```python
from build123d import *

# Parameters (mm, degrees)
F0_R     = 15.9266250138
F0_R_2   = 6.35
F1_DEPTH = 50.8
F2_R     = 3.4266006547
F3_DEPTH = 50.8
F7_R     = 6.4098114124
F8_DEPTH = 76.2


with BuildPart() as f1:
    # F0 (on Top) → F1 (new body)
    with BuildSketch(Plane.XY):
        Circle(F0_R)
        Circle(F0_R_2, mode=Mode.SUBTRACT)
    extrude(amount=F1_DEPTH)



with BuildPart() as f3:
    # F2 (on Top) → F3 (new body)
    with BuildSketch(Plane.XY):
        with Locations((-12.2786890715, 12.5171002001)):
            Circle(F2_R)
    extrude(amount=F3_DEPTH)


with BuildPart() as f4_1:
    # F4: copy of F3
    add(f3.part.moved(Location((24.45152, 0, 0))))


with BuildPart() as f5_1:
    # F5: copy of F4_1
    add(f4_1.part.moved(Location((0, -25.53886, 0))))


with BuildPart() as f6_1:
    # F6: copy of F5_1
    add(f5_1.part.moved(Location((-24.98095, 1.38116, 0))))


with BuildPart() as f1_1:
    add(f1.part)

    add(f3.part)  # F8 merges F3

    add(f4_1.part)  # F8 merges F4_1

    add(f5_1.part)  # F8 merges F5_1

    add(f6_1.part)  # F8 merges F6_1
    # F7 (on Top) → F8 (join, symmetric)
    with BuildSketch(Plane.XY):
        Circle(F7_R)
    extrude(amount=F8_DEPTH, both=True)


solid = f1_1.part
```
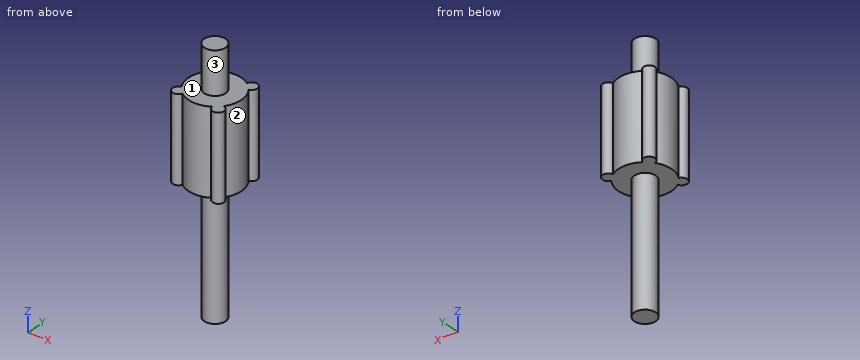
Build history of the part. All positions in model axes, mm. Face numbers are marked on the shaded views. Give positions to 0.01 mm unless a question says otherwise; leave off trailing zeros. Loops run counter-clockwise (first coordinate to the right, second up) from the corner with the lowest first, then second, coordinate; pieces in that order, holes last. Notation, with made-up numbers: (-22.5, 35.5) - (24.5, 35.5) arc R30 cw to (24.5, 68.5) - close; hole circle Ø7 at (45, 80.5). An arc over 180 degrees is marked (long way). Use a Markdown table: item, result.
(1) Band-saw the part on A-A (y = 0). Give the cut face in (x, z), and give its area (3 significant figures).
Taken from the geometry:
| item | result |
|---|---|
| outline | (-15.93, 0) - (-6.41, 0) - (-6.41, -76.2) - (6.41, -76.2) - (6.41, 0) - (15.93, 0) - (15.93, 50.8) - (6.41, 50.8) - (6.41, 76.2) - (-6.41, 76.2) - (-6.41, 50.8) - (-15.93, 50.8) - close |
| area | 2,920 mm2 |
(2) Band-saw the part on D-D (z = -9.5). Give the cut face in (x, y).
Taken from the geometry:
| item | result |
|---|---|
| outline | circle Ø12.82 at (0, 0) |
(3) Drop flat-ended pins along their axis: pin 1 Ø2 at (y, z) = (8.5, 5) entering from +X; pin 2 Ø3 at (x, z) = (-9.5, -57) entering from -Y; pin 3 Ø3 at (x, z) = (-3, -2) entering from -Y; pin 4 Ø10 at (x, z) = (-3.5, 19) entering from +Y. Give the stop position or say it passes through.
Taken from the geometry:
| item | result |
|---|---|
| pin 1 | x = 14.05 |
| pin 2 | through |
| pin 3 | y = -6.23 |
| pin 4 | y = 15.93 |
(4) Pull direction Y, two halves, no side cores. Call the marked faces 1, 2 and 3: +Y half, -Y half, draft (parallel to the pull), parting line (faces both ways), or undercut.
Taken from the geometry:
| item | result |
|---|---|
| face 1 | draft |
| face 2 | undercut |
| face 3 | parting line |
(5) Band-saw the part on C-C (z = 27). Give the cut face in (x, y), and give its area (3 significant figures).
Taken from the geometry:
| item | result |
|---|---|
| outline | (-13.59, -8.3) arc R3.43 ccw (long way) to (-9.56, -12.74) arc R15.93 ccw to (8.76, -13.3) arc R3.43 ccw (long way) to (12.68, -9.63) arc R15.93 ccw to (13.01, 9.19) arc R3.43 ccw (long way) to (8.83, 13.26) arc R15.93 ccw to (-8.92, 13.19) arc R3.43 ccw (long way) to (-13.02, 9.17) arc R15.93 ccw to start |
| area | 915 mm2 |
(6) Wall check: line 1 along Z through (x, y) = (-8.5, 11); line 2 along X through (y, z) = (10.5, 32.5); line 3 along Y through (x, z) = (-0.5, 8). Give the ranges that are in metal, low to high.
Taken from the geometry:
| item | result |
|---|---|
| line 1 | 0 to 50.8 |
| line 2 | -15.05 to 14.94 |
| line 3 | -15.92 to 15.92 |
